The model under review builds one solid part; all positions refer to its coordinate system, in mm. Face numbers are marked on the shaded views. A direction names the side the tool comes from. Give positions to 0.01 mm unless a question says otherwise; leave off trailing zeros. Order: outer loops, then holes, each group sorted by start corner. A loop starts at its lowest first (then second) coordinate and runs counter-clockwise, first axis right, second up. Notation, with made-up numbers: (30.5, 49) - (77.5, 49) arc R10 ccw to (77.5, 59) - close; hole circle Ø3 at (-28.75, -30.5). An arc over 180 degrees is marked (long way). Write item = value, one per line. Start each with the question number.
1. We need section B-B, the plane z = 3.75. Give the boundary of the cut face in (x, y), and give its area (3 significant figures).
2. We need section D-D, the plane y = 1.25. State how many separate pieces and enclosed holes the cut face has, and give its area (3 significant figures).
3. We need section C-C, the plane x = 2.5. Give the boundary of the cut face in (y, z).
4. We need section A-A, the plane x = 8. Give the boundary of the cut face in (y, z).
5. Machinability: for the marked faces 1 and 2, which of the approach directions +Z, -Z, +X, -X, +Y, -Y give a long, thin tool a straight path to every point of the face, cutting with its end or side? Answer none if there is none.
6. For P1, Ø0.7, axis at x = 25.5, z = -0.5, coming from the -Y side; P2, Ø0.7, axis at y = -2, z = 0.5, coming from the -X side; P3, Ø1.8, axis at x = 26.5, y = 2.5, coming from the +Z side; P4, Ø2, axis at x = 14, y = 1.5, coming from the +Z side, all flat-tipped, find the tip position at first contact; note any pin that passes through.
7. Wall thickness on probe 1 along Y at (x, z) = (16, 1.15); probe 2 along Y at (x, z) = (21, -0.75); probe 3 along Z at (x, y) = (16.5, 3): over which ranges is each line inside the solid? List them lowest first.
8. Mouldability with a two-part tool opening along X and no side actions: class the marked faces 3, 4, 5 and 6 as pulls with the +X half, pulls with the -X half, needs draft (parallel to the pull), parting line crosses it, or undercut.
from build123d import *
from build123d.topology import SkipClean

# Parameters (mm, degrees)
SKETCH1_R            = 2.4
BEAM_DEPTH           = 2
AXLE_CUT_DEPTH       = 29.017494535
AXLE_CUT_DEPTH_BACK  = 29.017494535
SKETCH2_W            = 1.8
SKETCH2_H            = 1.8
SKETCH3_R            = 3.1
HOLE_SURROUND_DEPTH  = 1.25
CAVITY_CUT_DEPTH     = 1.4
FILLET2_R            = 0.5
FILLET2_OF_MIRROR2_R = 0.5
FILLET3_R            = 0.5
SKETCH5_R            = 2.5
EXTENSION_DEPTH      = 3.85


with BuildPart() as part:
    # Sketch1 → Beam (new, symmetric)
    with BuildSketch(Plane.XY):
        with BuildLine():
            Line((0, 3.7), (24, 3.7))
            ThreePointArc((24, 3.7), (27.7, 0), (24, -3.7))
            Line((24, -3.7), (0, -3.7))
            ThreePointArc((0, -3.7), (-3.7, 0), (0, 3.7))
        make_face()
        with Locations((8, 0)):
            Circle(SKETCH1_R, mode=Mode.SUBTRACT)
        with Locations((16, 0)):
            Circle(SKETCH1_R, mode=Mode.SUBTRACT)
    extrude(amount=BEAM_DEPTH, both=True)

    # Sketch2 → Axle Cut (cut, two sides: drawn at the far end of the back side and taken through both)
    with BuildSketch(Plane.XY.offset(-AXLE_CUT_DEPTH_BACK)):
        Rectangle(SKETCH2_W, SKETCH2_H)
        with BuildLine():
            Line((-2.224859546, -0.9), (-0.9, -0.9))
            Line((-0.9, -0.9), (-0.9, 0.9))
            Line((-0.9, 0.9), (-2.224859546, 0.9))
            ThreePointArc((-2.224859546, 0.9), (-2.355808026, 0.45844143), (-2.4, 0))
            ThreePointArc((-2.4, 0), (-2.355808026, -0.45844143), (-2.224859546, -0.9))
        make_face()
        with BuildLine():
            Line((-0.9, 2.224859546), (-0.9, 0.9))
            Line((-0.9, 0.9), (0.9, 0.9))
            Line((0.9, 0.9), (0.9, 2.224859546))
            ThreePointArc((0.9, 2.224859546), (0.45844143, 2.355808026), (0, 2.4))
            ThreePointArc((0, 2.4), (-0.45844143, 2.355808026), (-0.9, 2.224859546))
        make_face()
        with BuildLine():
            Line((0.9, 0.9), (0.9, -0.9))
            Line((0.9, -0.9), (2.224859546, -0.9))
            ThreePointArc((2.224859546, -0.9), (2.355808026, -0.45844143), (2.4, 0))
            ThreePointArc((2.4, 0), (2.355808026, 0.45844143), (2.224859546, 0.9))
            Line((2.224859546, 0.9), (0.9, 0.9))
        make_face()
        with BuildLine():
            ThreePointArc((-0.9, -2.224859546), (-0.45844143, -2.355808026), (0, -2.4))
            ThreePointArc((0, -2.4), (0.45844143, -2.355808026), (0.9, -2.224859546))
            Line((0.9, -2.224859546), (0.9, -0.9))
            Line((0.9, -0.9), (-0.9, -0.9))
            Line((-0.9, -0.9), (-0.9, -2.224859546))
        make_face()
        with BuildLine():
            ThreePointArc((3.7, 0), (3.672112828, -0.453417441), (3.588871689, -0.9))
            ThreePointArc((3.588871689, -0.9), (3.188981578, -1.876271967), (2.529822128, -2.7))
            Line((2.529822128, -2.7), (5.470177872, -2.7))
            ThreePointArc((5.470177872, -2.7), (4.3, 0), (5.470177872, 2.7))
            Line((5.470177872, 2.7), (2.529822128, 2.7))
            ThreePointArc((2.529822128, 2.7), (3.188981578, 1.876271967), (3.588871689, 0.9))
            ThreePointArc((3.588871689, 0.9), (3.672112828, 0.453417441), (3.7, 0))
        make_face()
        with BuildLine():
            Line((2.4, 0), (2.4, -0.9))
            Line((2.4, -0.9), (3.588871689, -0.9))
            ThreePointArc((3.588871689, -0.9), (3.672112828, -0.453417441), (3.7, 0))
            ThreePointArc((3.7, 0), (3.672112828, 0.453417441), (3.588871689, 0.9))
            Line((3.588871689, 0.9), (2.4, 0.9))
            Line((2.4, 0.9), (2.4, 0))
        make_face()
        with BuildLine():
            ThreePointArc((2.224859546, 0.9), (2.355808026, 0.45844143), (2.4, 0))
            Line((2.4, 0), (2.4, 0.9))
            Line((2.4, 0.9), (2.224859546, 0.9))
        make_face()
        with BuildLine():
            ThreePointArc((2.4, 0), (2.355808026, -0.45844143), (2.224859546, -0.9))
            Line((2.224859546, -0.9), (2.4, -0.9))
            Line((2.4, -0.9), (2.4, 0))
        make_face()
        with BuildLine():
            Line((23.1, 2.224859546), (23.1, 0.9))
            Line((23.1, 0.9), (24.9, 0.9))
            Line((24.9, 0.9), (24.9, 2.224859546))
            ThreePointArc((24.9, 2.224859546), (24.45844143, 2.355808026), (24, 2.4))
            ThreePointArc((24, 2.4), (23.54155857, 2.355808026), (23.1, 2.224859546))
        make_face()
        with Locations((24, 0)):
            Rectangle(SKETCH2_W, SKETCH2_H)
        with BuildLine():
            ThreePointArc((21.775140454, 0.9), (21.644191974, 0.45844143), (21.6, 0))
            ThreePointArc((21.6, 0), (21.644191974, -0.45844143), (21.775140454, -0.9))
            Line((21.775140454, -0.9), (23.1, -0.9))
            Line((23.1, -0.9), (23.1, 0.9))
            Line((23.1, 0.9), (21.775140454, 0.9))
        make_face()
        with BuildLine():
            Line((24.9, -0.9), (23.1, -0.9))
            Line((23.1, -0.9), (23.1, -2.224859546))
            ThreePointArc((23.1, -2.224859546), (23.54155857, -2.355808026), (24, -2.4))
            ThreePointArc((24, -2.4), (24.45844143, -2.355808026), (24.9, -2.224859546))
            Line((24.9, -2.224859546), (24.9, -0.9))
        make_face()
        with BuildLine():
            Line((24.9, 0.9), (24.9, -0.9))
            Line((24.9, -0.9), (26.224859546, -0.9))
            ThreePointArc((26.224859546, -0.9), (26.355808026, -0.45844143), (26.4, 0))
            ThreePointArc((26.4, 0), (26.355808026, 0.45844143), (26.224859546, 0.9))
            Line((26.224859546, 0.9), (24.9, 0.9))
        make_face()
        with BuildLine():
            ThreePointArc((20.411128311, 0.9), (20.3, 0), (20.411128311, -0.9))
            Line((20.411128311, -0.9), (21.6, -0.9))
            Line((21.6, -0.9), (21.6, 0))
            Line((21.6, 0), (21.6, 0.9))
            Line((21.6, 0.9), (20.411128311, 0.9))
        make_face()
        with BuildLine():
            ThreePointArc((19.7, 0), (19.394874215, -1.471335809), (18.529822128, -2.7))
            Line((18.529822128, -2.7), (21.470177872, -2.7))
            ThreePointArc((21.470177872, -2.7), (20.811018422, -1.876271967), (20.411128311, -0.9))
            ThreePointArc((20.411128311, -0.9), (20.3, 0), (20.411128311, 0.9))
            ThreePointArc((20.411128311, 0.9), (20.811018422, 1.876271967), (21.470177872, 2.7))
            Line((21.470177872, 2.7), (18.529822128, 2.7))
            ThreePointArc((18.529822128, 2.7), (19.394874215, 1.471335809), (19.7, 0))
        make_face()
        with BuildLine():
            Line((21.6, 0), (21.6, -0.9))
            Line((21.6, -0.9), (21.775140454, -0.9))
            ThreePointArc((21.775140454, -0.9), (21.644191974, -0.45844143), (21.6, 0))
        make_face()
        with BuildLine():
            Line((21.6, 0.9), (21.6, 0))
            ThreePointArc((21.6, 0), (21.644191974, 0.45844143), (21.775140454, 0.9))
            Line((21.775140454, 0.9), (21.6, 0.9))
        make_face()
    extrude(amount=AXLE_CUT_DEPTH + AXLE_CUT_DEPTH_BACK, mode=Mode.SUBTRACT)

    # Sketch3 → Hole Surround (cut)
    with BuildSketch(Plane.XY.offset(2)):
        with Locations((16, 0)):
            Circle(SKETCH3_R)
        with Locations((8, 0)):
            Circle(SKETCH3_R)
    hole_surround = extrude(amount=-HOLE_SURROUND_DEPTH, mode=Mode.SUBTRACT)

    # Sketch4 → Cavity Cut (cut)
    with BuildSketch(Plane.XY.offset(2)):
        with BuildLine():
            Line((13.543885182, 2.7), (10.456114818, 2.7))
            ThreePointArc((10.456114818, 2.7), (11.338212028, 1.476089583), (11.65, 0))
            ThreePointArc((11.65, 0), (11.338212028, -1.476089583), (10.456114818, -2.7))
            Line((10.456114818, -2.7), (13.543885182, -2.7))
            ThreePointArc((13.543885182, -2.7), (12.35, 0), (13.543885182, 2.7))
        make_face()
    cavity_cut = extrude(amount=-CAVITY_CUT_DEPTH, mode=Mode.SUBTRACT)

    # Fillet2
    fillet2_edges = [part.edges().sort_by_distance(p)[0] for p in [
        (10.456114818, -2.7, 1.3),
        (10.456114818, 2.7, 1.3),
        (13.543885182, 2.7, 1.3),
        (13.543885182, -2.7, 1.3),
    ]]
    fillet(fillet2_edges, radius=FILLET2_R)

    # Mirror2: Hole Surround, Cavity Cut across plane
    add(hole_surround.mirror(Plane.XY), mode=Mode.SUBTRACT)
    add(cavity_cut.mirror(Plane.XY), mode=Mode.SUBTRACT)

    # Fillet2 of Mirror2
    fillet2_of_mirror2_edges = [part.edges().sort_by_distance(p)[0] for p in [
        (10.456114818, -2.7, -1.3),
        (10.456114818, 2.7, -1.3),
        (13.543885182, 2.7, -1.3),
        (13.543885182, -2.7, -1.3),
    ]]
    fillet(fillet2_of_mirror2_edges, radius=FILLET2_OF_MIRROR2_R)

    # Fillet3
    fillet3_edges = [part.edges().sort_by_distance(p)[0] for p in [
        (2.529822128, 2.7, 0),
        (5.470177872, 2.7, 0),
        (5.470177872, -2.7, 0),
        (2.529822128, -2.7, 0),
        (21.470177872, -2.7, 0),
        (18.529822128, -2.7, 0),
        (18.529822128, 2.7, 0),
        (21.470177872, 2.7, 0),
    ]]
    fillet(fillet3_edges, radius=FILLET3_R)

    # Sketch5 → Extension (add)
    with SkipClean():  # the faces are left unmerged after this step: merging them gives an invalid solid
        with BuildSketch(Plane.XY.offset(2)):
            with BuildLine():
                ThreePointArc((27.299887499, -1.673541902), (27.7, 0), (27.299887499, 1.673541902))
                ThreePointArc((27.299887499, 1.673541902), (26.2627417, 2.2627417), (25.673541902, 3.299887499))
                ThreePointArc((25.673541902, 3.299887499), (24, 3.7), (22.326458098, 3.299887499))
                ThreePointArc((22.326458098, 3.299887499), (21.7372583, 2.2627417), (20.700112501, 1.673541902))
                ThreePointArc((20.700112501, 1.673541902), (20.3, 0), (20.700112501, -1.673541902))
                ThreePointArc((20.700112501, -1.673541902), (21.7372583, -2.2627417), (22.326458098, -3.299887499))
                ThreePointArc((22.326458098, -3.299887499), (24, -3.7), (25.673541902, -3.299887499))
                ThreePointArc((25.673541902, -3.299887499), (26.2627417, -2.2627417), (27.299887499, -1.673541902))
            make_face()
            with Locations(Location((24, 0, 0), (0, 0, 201.100196024))):
                Circle(SKETCH5_R, mode=Mode.SUBTRACT)
        extrude(amount=EXTENSION_DEPTH)


solid = part.part
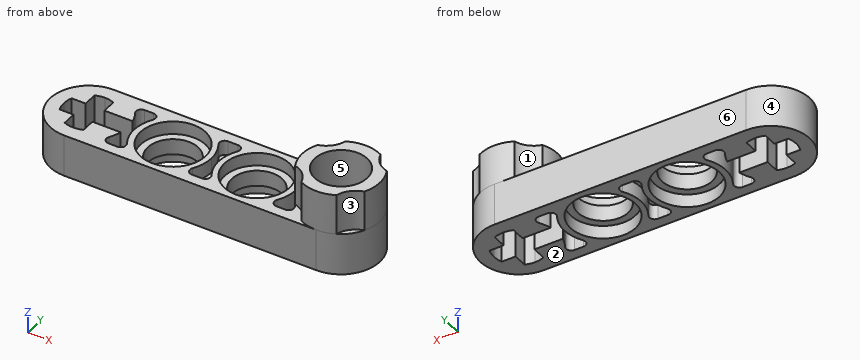
Model answer:
q1.outline = (20.7, -1.67) arc R2.25 cw to (22.33, -3.3) arc R3.7 ccw to (25.67, -3.3) arc R2.25 cw to (27.3, -1.67) arc R3.7 ccw to (27.3, 1.67) arc R2.25 cw to (25.67, 3.3) arc R3.7 ccw to (22.33, 3.3) arc R2.25 cw to (20.7, 1.67) arc R3.7 ccw to start; hole circle Ø5 at (24, 0)
q1.area = 20.3 mm2
q2.separate_pieces = 7
q2.enclosed_holes = 0
q2.area = 67.5 mm2
q3.outline = (-3.7, -2) - (-0.9, -2) - (-0.9, 2) - (-3.7, 2) - close; (0.9, -2) - (3.7, -2) - (3.7, 2) - (0.9, 2) - close
q4.outline = (-3.7, -2) - (-3.1, -2) - (-3.1, -0.75) - (-2.4, -0.75) - (-2.4, 0.75) - (-3.1, 0.75) - (-3.1, 2) - (-3.7, 2) - close; (2.4, -0.75) - (3.1, -0.75) - (3.1, -2) - (3.7, -2) - (3.7, 2) - (3.1, 2) - (3.1, 0.75) - (2.4, 0.75) - close
q5.face_1 = +Z, -X, +Y
q5.face_2 = -Z, +X, -X, +Y, -Y
q6.P1 = -3.52
q6.P2 = -3.31
q6.P3 = 5.85
q6.P4 = 2
q7.probe_1 = -3.7 to -3.1, 3.1 to 3.7
q7.probe_2 = -3.7 to -0.9, 0.9 to 3.7
q7.probe_3 = -0.75 to 0.75
q8.face_3 = pulls with the +X half
q8.face_4 = pulls with the -X half
q8.face_5 = undercut
q8.face_6 = needs draft
